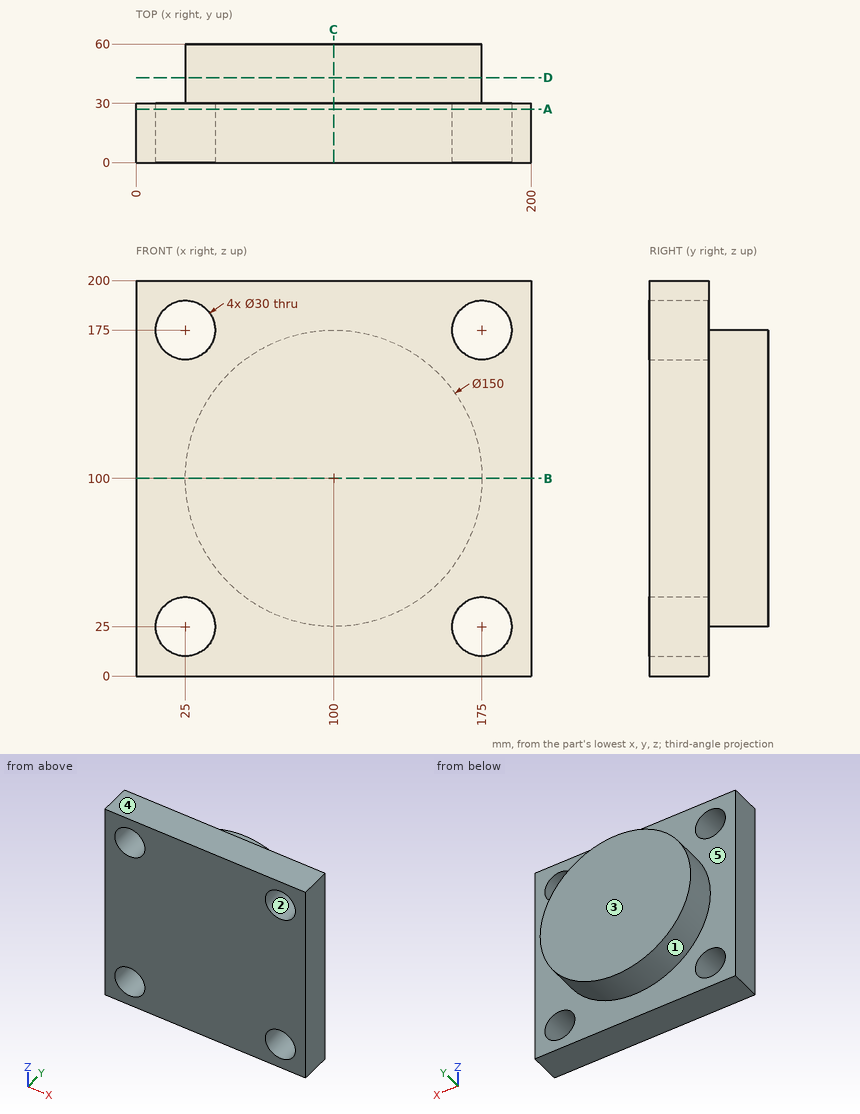
For this review, use the dimensioned drawing (mm, ordinates from the lowest corner) and the shaded views. A direction names the side the tool comes from. Round coordinates to 2 decimals unless told otherwise and drop trailing zeros. Write each loop counter-clockwise with the first axis right and the second up, starting at its lowest first coordinate (ties: lowest second). Pieces come first, ordered by that corner, then holes. Notation, with made-up numbers: M -23,85.5 L -5,85.5 A27 cw -5,118.5 Z; hole C -5,-3.5 d4. An arc over 180 degrees is marked long. Use CSV: the item, a comma, the result in double quotes. Start each with the question number.
(1) We need section D-D, the plane y = 43. State the section outline as (x, z) points.
(2) We need section A-A, the plane y = 27. State the section outline as (x, z) points, then the cut area to 3 significant figures.
(3) The part is to be moulded in two halves that separate along Z. For the marked faces 1, 2 and 3, say which applies: +Z half, -Z half, draft (parallel to the pull), parting line (faces both ways), or undercut.
(4) Tool access review of the marked faces 4 and 5: name each direction out of +Z, -Z, +X, -X, +Y, -Y from which nothing blocks a thin tool from reaching the whole face with its end or side.
(5) Clearance check with flat-ended pins moving along their axes: P1, Ø4, axis at x = 144, y = 41, coming from the +Z side; P2, Ø1, axis at y = 41, z = 60, coming from the -X side. State where each tip first meets the part, or that it passes through.
(6) For line 1 along X through (y, z) = (12.25, 25); line 2 along Z through (x, y) = (34, 7.5), list the stretches that pass through material, from the lowest coordinate up.
(7) We need section C-C, the plane x = 100. State the section outline as (y, z) points, then the cut area to 3 significant figures.
(8) We need section B-B, the plane z = 100. State the section outline as (x, y) points.
Findings:
1,outline,"C 100,100 d150"
2,outline,"M 0,0 L 200,0 L 200,200 L 0,200 Z; hole C 25,25 d30; hole C 25,175 d30; hole C 175,25 d30; hole C 175,175 d30"
2,area,"37,200 mm^2"
3,face 1,"parting line"
3,face 2,"undercut"
3,face 3,"draft"
4,face 4,"+Z, +X, -X, +Y, -Y"
4,face 5,"+Y"
5,P1,"z = 162.14"
5,P2,"x = 36.24"
6,line 1,"0 to 10, 40 to 160, 190 to 200"
6,line 2,"0 to 13, 37 to 163, 187 to 200"
7,outline,"M 0,0 L 30,0 L 30,25 L 60,25 L 60,175 L 30,175 L 30,200 L 0,200 Z"
7,area,"10,500 mm^2"
8,outline,"M 0,0 L 200,0 L 200,30 L 175,30 L 175,60 L 25,60 L 25,30 L 0,30 Z"
